```python
from build123d import *

# Parameters (mm, degrees)
SKETCH1_W                = 19
SKETCH1_H                = 19
SKETCH1_W_2              = 12.12
SKETCH1_H_2              = 12.12
BOSS_EXTRUDE1_DEPTH      = 20
SKETCH2_R                = 1.55
CUT_EXTRUDE1_DEPTH       = 22
SKETCH3_W                = 12.92
SKETCH3_H                = 12.92
CUT_EXTRUDE2_DEPTH       = 20
BOSS_EXTRUDE2_DEPTH      = 40
BOSS_EXTRUDE2_DEPTH_BACK = 3.04
CUT_EXTRUDE3_DEPTH       = 40
SKETCH7_W                = 13
SKETCH7_H                = 3
BOSS_EXTRUDE3_DEPTH      = 30
CUT_EXTRUDE4_DEPTH       = 129
FILLET2_R                = 3
FILLET3_R                = 3
FILLET4_R                = 3
FILLET5_SIZE             = 4.75
FILLET6_SIZE             = 3
FILLET7_SIZE             = 3
FILLET8_SIZE             = 1


with BuildPart() as part:
    # Sketch1 → Boss-Extrude1 (new body)
    with BuildSketch(Plane(origin=(0, 0, 0), x_dir=(1, 0, 0), z_dir=(0, 1, 0))):
        with Locations((9.5, 9.5)):
            Rectangle(SKETCH1_W, SKETCH1_H)
        with Locations((9.5, 9.5)):
            Rectangle(SKETCH1_W_2, SKETCH1_H_2, mode=Mode.SUBTRACT)
    extrude(amount=BOSS_EXTRUDE1_DEPTH)

    # Sketch2 → Cut-Extrude1 (cut)
    with BuildSketch(Plane.XY):
        with Locations((9.5, 16)):
            Circle(SKETCH2_R)
        with Locations((9.5, 3.5)):
            Circle(SKETCH2_R)
    extrude(amount=-CUT_EXTRUDE1_DEPTH, mode=Mode.SUBTRACT)

    # Sketch3 → Cut-Extrude2 (cut)
    with BuildSketch(Plane.XZ):
        with Locations((9.5, -9.5)):
            Rectangle(SKETCH3_W, SKETCH3_H)
    extrude(amount=-CUT_EXTRUDE2_DEPTH, mode=Mode.SUBTRACT)

    # Sketch4 → Boss-Extrude2 (add, two sides: drawn at the far end of the back side and taken through both)
    with BuildSketch(Plane.ZY.offset(-BOSS_EXTRUDE2_DEPTH_BACK)):
        Polygon((-11, 70), (-11, -4.746484506), (-8, -4.746484506), (-8, 70), (-8, 85), (-11, 85), align=None)
    extrude(amount=BOSS_EXTRUDE2_DEPTH + BOSS_EXTRUDE2_DEPTH_BACK)

    # Sketch5 → Cut-Extrude3 (cut)
    with BuildSketch(Plane.XY.offset(-8)):
        Polygon((-16.96, 85), (3.04, 20), (3.04, 85), align=None)
    extrude(amount=-CUT_EXTRUDE3_DEPTH, mode=Mode.SUBTRACT)

    # Sketch7 → Boss-Extrude3 (add)
    with BuildSketch(Plane.XZ.offset(4.746484506)):
        with Locations((-33.5, -9.5)):
            Rectangle(SKETCH7_W, SKETCH7_H)
    extrude(amount=BOSS_EXTRUDE3_DEPTH)

    # Sketch8 → Cut-Extrude4 (cut)
    with BuildSketch(Plane.XZ.offset(34.746484506)):
        Polygon((-40, -8), (-40, -9.5), (-36.5, -8), align=None)
        Polygon((-36.5, -11), (-40, -9.5), (-40, -11), align=None)
    extrude(amount=-CUT_EXTRUDE4_DEPTH, mode=Mode.SUBTRACT)

    # Fillet2
    fillet2_edges = [part.edges().sort_by_distance(p)[0] for p in [
        (-27, -4.746484506, -9.5),
    ]]
    fillet(fillet2_edges, radius=FILLET2_R)

    # Fillet3
    fillet3_edges = [part.edges().sort_by_distance(p)[0] for p in [
        (-27, -34.746484506, -9.5),
    ]]
    fillet(fillet3_edges, radius=FILLET3_R)

    # Fillet4
    fillet4_edges = [part.edges().sort_by_distance(p)[0] for p in [
        (-16.96, 85, -9.5),
    ]]
    fillet(fillet4_edges, radius=FILLET4_R)

    # Fillet5
    # the kernel refuses this chamfer: 4.75 mm, written as the material it adds along each edge
    with BuildSketch(Plane(origin=(3.04, 0, -8), x_dir=(0, -0.9996219169112968, -0.027495876610586535), z_dir=(-1, 0, 0))) as fillet5_piece_1_section:
        Polygon((FILLET5_SIZE * 0.999621916911, FILLET5_SIZE * 0.0274958766106), (-FILLET5_SIZE * 0.0274958766106, FILLET5_SIZE * 0.999621916911), (0, 0), align=None)
    fillet5_piece_1 = extrude(amount=3.04, mode=Mode.PRIVATE)
    fillet5_piece_1 = split(fillet5_piece_1, bisect_by=Plane(origin=(1.52, -4.746484506, -6.430475531), z_dir=(0, 1, 0)), keep=Keep.TOP, mode=Mode.PRIVATE)
    add(fillet5_piece_1)
    with BuildSketch(Plane(origin=(0, 0, -11), x_dir=(0, 0.02749587661058637, -0.9996219169112968), z_dir=(1, 0, 0))) as fillet5_piece_2_section:
        Polygon((FILLET5_SIZE * 0.999621916911, -FILLET5_SIZE * 0.0274958766106), (-FILLET5_SIZE * 0.0274958766106, -FILLET5_SIZE * 0.999621916911), (0, 0), align=None)
    fillet5_piece_2 = extrude(amount=3.04, mode=Mode.PRIVATE)
    fillet5_piece_2 = split(fillet5_piece_2, bisect_by=Plane(origin=(1.52, -4.746484506, -12.569524469), z_dir=(0, 1, 0)), keep=Keep.TOP, mode=Mode.PRIVATE)
    add(fillet5_piece_2)

    # Fillet6
    fillet6_edges = [part.edges().sort_by_distance(p)[0] for p in [
        (1.52, 20, -11),
        (1.52, 20, -8),
    ]]
    chamfer(fillet6_edges, length=FILLET6_SIZE)

    # Fillet7
    fillet7_edges = [part.edges().sort_by_distance(p)[0] for p in [
        (0, 9.126757747, -11),
        (0, 9.126757747, -8),
    ]]
    chamfer(fillet7_edges, length=FILLET7_SIZE)

    # Fillet8
    fillet8_edges = [part.edges().sort_by_distance(p)[0] for p in [
        (0, 10, -19),
        (19, 10, -19),
        (19, 10, 0),
        (0, 10, 0),
    ]]
    chamfer(fillet8_edges, length=FILLET8_SIZE)


solid = part.part
```
Check sheet for the modelled part. Datum: model origin and axes. Units: mm. A direction names the side the tool comes from. Coordinates: 2 decimals unless noted, no trailing zeros. Order: outer loops, then holes, each group sorted by start corner. A loop starts at its lowest first (then second) coordinate and runs counter-clockwise, first axis right, second up. Notation, with made-up numbers: (-21, 45.25) -> (13, 45.25) arc R14 ccw to (13, 56.25) -> close; hole circle Ø1 at (46.25, 79.25). An arc over 180 degrees is marked (long way). Write item = value, one per line. Start each with the question number.
1) Cross-section at C-C (y = 48). Enter the section's corners in (x, z), then the cut area to 3 significant figures.
2) Cross-section at D-D (y = 77). Enter the section's corners in (x, z), then the cut area to 3 significant figures.
3) Go/stop test with flat-tipped pins: P1, Ø8, axis at x = -21.5, y = 39, coming from the -Z side; P2, Ø2.5, axis at x = -9.5, z = -9.5, coming from the -Y side; P3, Ø5, axis at x = 9.5, y = 3.5, coming from the -Z side; P4, Ø2, axis at y = 14, z = -2.5, coming from the -X side. Record where each tip stops, or that it passes through.
4) Mould release check, pull along X, two halves, no side actions. Record for faces 1 (the flat face through (-2, 9, -7)), 2 (the flat face through (9, 10, -19)), 3 (the cylindrical face through (8.27, 2.56, -17.46)), 4 (the cylindrical face through (-26.145, -5.649, -9.479)): +X half, -X half, draft (parallel to the pull), parting line (faces both ways), or undercut.
5) Access from +Z, -Z, +X, -X, +Y, -Y to the whole of each face (thin tool, end or side, straight path). Record for faces 5 (the flat face through (3.04, 8, -10)), 6 (the cylindrical face through (-17.415, 84.429, -9.521)), 7 (the flat face through (0, 9, -3)).
6) Cross-section at B-B (x = 9.5). Enter the section's corners in (y, z), then the cut area to 3 significant figures.
7) Cross-section at A-A (y = 3.5). Enter the section's corners in (x, z), then the cut area to 3 significant figures.
8) Material ranges on L1, parallel to Y at x = 9.5, z = -18.1; L2, parallel to Z at x = -28.5, y = -18; L3, parallel to Y at x = -19, z = -8.75, recorded low to high.
Ans:
q1.outline = (-40, -9.5) -> (-36.5, -11) -> (-5.58, -11) -> (-5.58, -8) -> (-36.5, -8) -> close
q1.area = 98.0 mm²
q2.outline = (-40, -9.5) -> (-36.5, -11) -> (-14.5, -11) -> (-14.5, -8) -> (-36.5, -8) -> close
q2.area = 71.3 mm²
q3.P1 = -11
q3.P2 = -4.75
q3.P3 = -19
q3.P4 = 0
q4.face_1 = -X half
q4.face_2 = draft
q4.face_3 = undercut
q4.face_4 = +X half
q5.face_5 = +Y, -Y
q5.face_6 = +Z, -Z, +X, +Y
q5.face_7 = +Z, -X, +Y, -Y
q6.outline = (0, -19) -> (1.95, -19) -> (1.95, -15.96) -> (0, -15.96) -> close; (0, -3.04) -> (1.95, -3.04) -> (1.95, 0) -> (0, 0) -> close; (5.05, -19) -> (14.45, -19) -> (14.45, -15.96) -> (5.05, -15.96) -> close; (5.05, -3.04) -> (14.45, -3.04) -> (14.45, 0) -> (5.05, 0) -> close; (17.55, -19) -> (20, -19) -> (20, -15.96) -> (17.55, -15.96) -> close; (17.55, -3.04) -> (20, -3.04) -> (20, 0) -> (17.55, 0) -> close
q6.area = 83.9 mm²
q7.outline = (-40, -9.5) -> (-36.5, -11) -> (-3, -11) -> (0, -14) -> (0, -18) -> (1, -19) -> (7.95, -19) -> (7.95, -15.96) -> (3.04, -15.96) -> (3.04, -3.04) -> (7.95, -3.04) -> (7.95, 0) -> (1, 0) -> (0, -1) -> (0, -5) -> (-3, -8) -> (-36.5, -8) -> close; (11.05, -19) -> (18, -19) -> (19, -18) -> (19, -1) -> (18, 0) -> (11.05, 0) -> (11.05, -3.04) -> (15.96, -3.04) -> (15.96, -15.96) -> (11.05, -15.96) -> close
q7.area = 297 mm²
q8.L1 = 0 to 1.95, 5.05 to 14.45, 17.55 to 20
q8.L2 = -11 to -8
q8.L3 = -4.75 to 84.99
